Could you check a few things on this model? Use its own coordinates, in mm. A direction names the side the tool comes from. Coordinates: 2 decimals unless noted, no trailing zeros. Loops run counter-clockwise (first coordinate to the right, second up) from the corner with the lowest first, then second, coordinate; pieces in that order, holes last. Notation, with made-up numbers: (-9.75, 55.25) -> (45.25, 55.25) arc R6 ccw to (45.25, 61.25) -> close; hole circle Ø9 at (64.5, 52.5). An arc over 180 degrees is marked (long way). One line per question, with ' | ' between items.
from build123d import *

# Parameters (mm, degrees)
SKETCH2_R           = 60
SKETCH2_R_2         = 50
BOSS_EXTRUDE1_DEPTH = 5
SKETCH7_R           = 80
SKETCH7_R_2         = 50
BOSS_EXTRUDE2_DEPTH = 5
SKETCH8_R           = 80
SKETCH8_R_2         = 70
BOSS_EXTRUDE3_DEPTH = 22
CUT_EXTRUDE3_REACH  = 119.576
SKETCH4_R           = 2.5
SKETCH9_R           = 2.5
CUT_EXTRUDE4_DEPTH  = 10


with BuildPart() as part:
    # Sketch2 → Boss-Extrude1 (new body)
    with BuildSketch(Plane(origin=(0, 0, 0), x_dir=(1, 0, 0), z_dir=(0, 1, 0))):
        with Locations(Location((0, 0, 0), (0, 0, 270))):
            Circle(SKETCH2_R)
        with Locations(Location((0, 0, 0), (0, 0, 270))):
            Circle(SKETCH2_R_2, mode=Mode.SUBTRACT)
    extrude(amount=BOSS_EXTRUDE1_DEPTH)

    # Sketch7 → Boss-Extrude2 (add)
    with BuildSketch(Plane(origin=(0, 5, 0), x_dir=(1, 0, 0), z_dir=(0, 1, 0))):
        with Locations(Location((0, 0, 0), (0, 0, 270))):
            Circle(SKETCH7_R)
        with Locations(Location((0, 0, 0), (0, 0, 270))):
            Circle(SKETCH7_R_2, mode=Mode.SUBTRACT)
    extrude(amount=BOSS_EXTRUDE2_DEPTH)

    # Sketch8 → Boss-Extrude3 (add)
    with BuildSketch(Plane(origin=(0, 10, 0), x_dir=(1, 0, 0), z_dir=(0, 1, 0))):
        with Locations(Location((0, 0, 0), (0, 0, 270))):
            Circle(SKETCH8_R)
        with Locations(Location((0, 0, 0), (0, 0, 270))):
            Circle(SKETCH8_R_2, mode=Mode.SUBTRACT)
    extrude(amount=BOSS_EXTRUDE3_DEPTH)

    # Sketch4 → Cut-Extrude3 (cut, up to next)
    with BuildSketch(Plane.XZ, mode=Mode.PRIVATE) as cut_extrude3_sk1:
        with Locations(Location((-55, 0, 0), (0, 0, 270))):
            Circle(SKETCH4_R)
    cut_extrude3_tool1 = extrude(cut_extrude3_sk1.sketch, amount=-CUT_EXTRUDE3_REACH, mode=Mode.PRIVATE) & part.part
    # Sketch4 → Cut-Extrude3 (cut, up to next)
    with BuildSketch(Plane.XZ, mode=Mode.PRIVATE) as cut_extrude3_sk2:
        with Locations(Location((0, 55, 0), (0, 0, 270))):
            Circle(SKETCH4_R)
    cut_extrude3_tool2 = extrude(cut_extrude3_sk2.sketch, amount=-CUT_EXTRUDE3_REACH, mode=Mode.PRIVATE) & part.part
    # Sketch4 → Cut-Extrude3 (cut, up to next)
    with BuildSketch(Plane.XZ, mode=Mode.PRIVATE) as cut_extrude3_sk3:
        with Locations(Location((0, -55, 0), (0, 0, 270))):
            Circle(SKETCH4_R)
    cut_extrude3_tool3 = extrude(cut_extrude3_sk3.sketch, amount=-CUT_EXTRUDE3_REACH, mode=Mode.PRIVATE) & part.part
    # Sketch4 → Cut-Extrude3 (cut, up to next)
    with BuildSketch(Plane.XZ, mode=Mode.PRIVATE) as cut_extrude3_sk4:
        with Locations(Location((55, 0, 0), (0, 0, 270))):
            Circle(SKETCH4_R)
    cut_extrude3_tool4 = extrude(cut_extrude3_sk4.sketch, amount=-CUT_EXTRUDE3_REACH, mode=Mode.PRIVATE) & part.part
    add(cut_extrude3_tool1.solids().sort_by_distance((-55, 0, 0))[0], mode=Mode.SUBTRACT)
    add(cut_extrude3_tool2.solids().sort_by_distance((0, 0, 55))[0], mode=Mode.SUBTRACT)
    add(cut_extrude3_tool3.solids().sort_by_distance((0, 0, -55))[0], mode=Mode.SUBTRACT)
    add(cut_extrude3_tool4.solids().sort_by_distance((55, 0, 0))[0], mode=Mode.SUBTRACT)

    # Sketch9 → Cut-Extrude4 (cut)
    with BuildSketch(Plane(origin=(0, 32, 0), x_dir=(1, 0, 0), z_dir=(0, 1, 0))):
        with Locations(Location((-75, 0, 0), (0, 0, 270))):
            Circle(SKETCH9_R)
        with Locations(Location((0, 75, 0), (0, 0, 270))):
            Circle(SKETCH9_R)
        with Locations(Location((0, -75, 0), (0, 0, 270))):
            Circle(SKETCH9_R)
        with Locations(Location((75, 0, 0), (0, 0, 270))):
            Circle(SKETCH9_R)
    extrude(amount=-CUT_EXTRUDE4_DEPTH, mode=Mode.SUBTRACT)


solid = part.part
1) If we section it at C-C on x = -43: Please give me the cut outline in (y, z), and give its area (3 significant figures).
Data:
outline: (0, -41.84) -> (5, -41.84) -> (5, -67.46) -> (32, -67.46) -> (32, -55.24) -> (10, -55.24) -> (10, -25.51) -> (0, -25.51) -> close; (0, 25.51) -> (10, 25.51) -> (10, 55.24) -> (32, 55.24) -> (32, 67.46) -> (5, 67.46) -> (5, 41.84) -> (0, 41.84) -> close | area: 1,120 mm²
2) I'm going to push flat-ended pins straight in: pin 1 Ø6.5 at (x, z) = (0, -55) entering from +Y; pin 2 Ø4 at (x, z) = (0, -75) entering from +Y; pin 3 Ø5 at (x, y) = (-41.5, 21) entering from +Z; pin 4 Ø5.5 at (x, z) = (-74.5, 1) entering from +Y. Where does each tip first touch, or does it pass through?
Data:
pin 1: y = 10 | pin 2: y = 22 | pin 3: z = 69.85 | pin 4: y = 32
3) If we section it at A-A on x = 0: Give the number of separate pieces and of enclosed holes in the cut face, and give its area (3 significant figures).
Data:
separate pieces: 4 | enclosed holes: 0 | area: 640 mm²
4) On a 3-axis mill with a long thin cutter (end or side, diameter ignored), from which of +Z, -Z, +X, -X, +Y, -Y can I reach the whole of each face in a straight line? I mean faces 4 (the face through (60, 5, 11)), 5 (the face through (17, 10, -48)), 6 (the face through (-0.96, 4.93, 52.69)). Say none if no direction works.
Data:
face 4: -Y | face 5: +Y | face 6: +Y, -Y
5) If we section it at D-D on z = -36: Please give me the cut outline in (x, y).
Data:
outline: (-71.44, 5) -> (-48, 5) -> (-48, 0) -> (-34.7, 0) -> (-34.7, 10) -> (-60.03, 10) -> (-60.03, 32) -> (-71.44, 32) -> close; (34.7, 0) -> (48, 0) -> (48, 5) -> (71.44, 5) -> (71.44, 32) -> (60.03, 32) -> (60.03, 10) -> (34.7, 10) -> close
6) We'd pull the mould along Z, two halves only. Please class faces 1 (the face through (0, 22, -75)), 2 (the face through (-78.1, 18.31, -17.34)), 3 (the face through (45, 0, -23)): pulls with the +Z half, pulls with the -Z half, needs draft (parallel to the pull), parting line crosses it, or undercut.
Data:
face 1: undercut | face 2: parting line crosses it | face 3: needs draft
7) I need wall thicknesses on line 1 along X through (y, z) = (24.5, 0); line 2 along X through (y, z) = (20, 0); line 3 along Y through (x, z) = (-50, -24.5). Which ranges of each line are inside material? Lowest first, please. Write a range as from..to.
Data:
line 1: -80..-77.5, -72.5..-70, 70..72.5, 77.5..80 | line 2: -80..-70, 70..80 | line 3: 0..10
